from build123d import *

# Parameters (mm, degrees)
F0_R     = 13.75
F1_DEPTH = 10
F2_R     = 478.617491


with BuildPart() as f1:
    # F0 (on Top) → F1 (new body)
    with BuildSketch(Plane.XY):
        with BuildLine():
            ThreePointArc((-84.117798, 27.214582), (-67.273856, 17.994112), (-60.569575, 0))
            ThreePointArc((-60.569575, 0), (-67.273856, -17.994112), (-84.117798, -27.214582))
            Line((-84.117798, -27.214582), (0, -15))
            Line((0, -15), (84.117798, -27.214582))
            ThreePointArc((84.117798, -27.214582), (60.569575, 0), (84.117798, 27.214582))
            Line((84.117798, 27.214582), (0, 15))
            Line((0, 15), (-84.117798, 27.214582))
        make_face()
        with BuildLine():
            ThreePointArc((-84.117798, -27.214582), (-67.273856, -17.994112), (-60.569575, 0))
            ThreePointArc((-60.569575, 0), (-67.273856, 17.994112), (-84.117798, 27.214582))
            ThreePointArc((-84.117798, 27.214582), (-115.569575, 0), (-84.117798, -27.214582))
        make_face()
        with Locations((-88.069575, 0)):
            Circle(F0_R, mode=Mode.SUBTRACT)
        with BuildLine():
            ThreePointArc((115.569575, 0), (106.063687, 20.795719), (84.117798, 27.214582))
            ThreePointArc((84.117798, 27.214582), (60.569575, 0), (84.117798, -27.214582))
            ThreePointArc((84.117798, -27.214582), (106.063687, -20.795719), (115.569575, 0))
        make_face()
        with Locations((88.069575, 0)):
            Circle(F0_R, mode=Mode.SUBTRACT)
    extrude(amount=F1_DEPTH)

    # F2
    f2_edges = [f1.edges().sort_by_distance(p)[0] for p in [
        (0, -15, 5),
        (0, 15, 5),
    ]]
    fillet(f2_edges, radius=F2_R)


solid = f1.part
The listing builds one solid part. Answer for the finished solid, in the listing's coordinates (mm). A direction names the side the tool comes from. Give positions to 0.01 mm unless a question says otherwise; leave off trailing zeros. Loops run counter-clockwise (first coordinate to the right, second up) from the corner with the lowest first, then second, coordinate; pieces in that order, holes last.
Item 1: A cutting plane is placed at B-B (x = -87). Give the vertices of the cut face in (y, z), then the cut area to 3 significant figures.
Derived:
outline: (-27.48, 0) - (-13.71, 0) - (-13.71, 10) - (-27.48, 10) - close; (13.71, 0) - (27.48, 0) - (27.48, 10) - (13.71, 10) - close
area: 275 mm2
Item 2: Each of these flat-tipped pins is pushed along its axis until it touches: pin 1 Ø16.5 at (x, y) = (-88.07, 0) entering from -Z; pin 2 Ø1.5 at (y, z) = (2.5, 1.5) entering from -X; pin 3 Ø3 at (x, z) = (51, 1) entering from +Y; pin 4 Ø4 at (y, z) = (11.5, 8) entering from +X. Where does it stop, or does it pass through?
Derived:
pin 1: passes through
pin 2: stops at x = -115.51
pin 3: stops at y = 22.91
pin 4: stops at x = 113.88
Item 3: Find the intervals of material crossed by line 1 along X through (y, z) = (-4.5, 8); line 2 along X through (y, z) = (-11, 5.5); line 3 along Y through (x, z) = (1, 9.5), in increasing order.
Derived:
line 1: x = -115.2 to -101.06, -75.08 to 75.08, 101.06 to 115.2
line 2: x = -113.27 to -96.32, -79.82 to 79.82, 96.32 to 113.27
line 3: y = -20.02 to 20.02
Item 4: A cutting plane is placed at D-D (y = -2.5). Give the vertices of the cut face in (x, z), then the cut area to 3 significant figures.
Derived:
outline: (-115.46, 0) - (-101.59, 0) - (-101.59, 10) - (-115.46, 10) - close; (-74.55, 0) - (74.55, 0) - (74.55, 10) - (-74.55, 10) - close; (101.59, 0) - (115.46, 0) - (115.46, 10) - (101.59, 10) - close
area: 1,770 mm2
Item 5: A cutting plane is placed at C-C (y = 11). Give the vertices of the cut face in (x, z).
Derived:
outline: (-113.27, 0) - (-96.32, 0) - (-96.32, 10) - (-113.27, 10) - close; (-79.82, 0) - (79.82, 0) - (79.82, 10) - (-79.82, 10) - close; (96.32, 0) - (113.27, 0) - (113.27, 10) - (96.32, 10) - close
Item 6: Determine the mould class of faces 1 (the flat face through (-76.34, 26.085, 4.93)), 2 (the flat face through (-2, 0, 0)) for opening direction X: +X half, -X half, draft (parallel to the pull), parting line (faces both ways), or undercut.
Derived:
face 1: undercut
face 2: draft
Item 7: A tool of negligible diameter and unlimited length cuts with its end or side. For faces 3 (the flat face through (-76.555, -26.116, 4.93)), 4 (the flat face through (76.555, 26.116, 4.93)), 5 (the cylindrical face through (77.16, -8.37, 4.93)), from which of +Z, -Z, +X, -X, +Y, -Y can it reach the whole face along a straight path? Write none if from no direction.
Derived:
face 3: +Z, -Z, -Y
face 4: +Z, -Z, +Y
face 5: +Z, -Z
Item 8: A cutting plane is placed at A-A (z = 6). Give the vertices of the cut face in (x, y).
Derived:
outline: (-84.12, -27.21) - (-68.78, -24.99) arc R478.62 cw to (68.78, -24.99) - (84.12, -27.21) arc R27.5 ccw (long way) to (84.12, 27.21) - (68.78, 24.99) arc R478.62 cw to (-68.78, 24.99) - (-84.12, 27.21) arc R27.5 ccw (long way) to start; hole circle Ø27.5 at (-88.07, 0); hole circle Ø27.5 at (88.07, 0)
